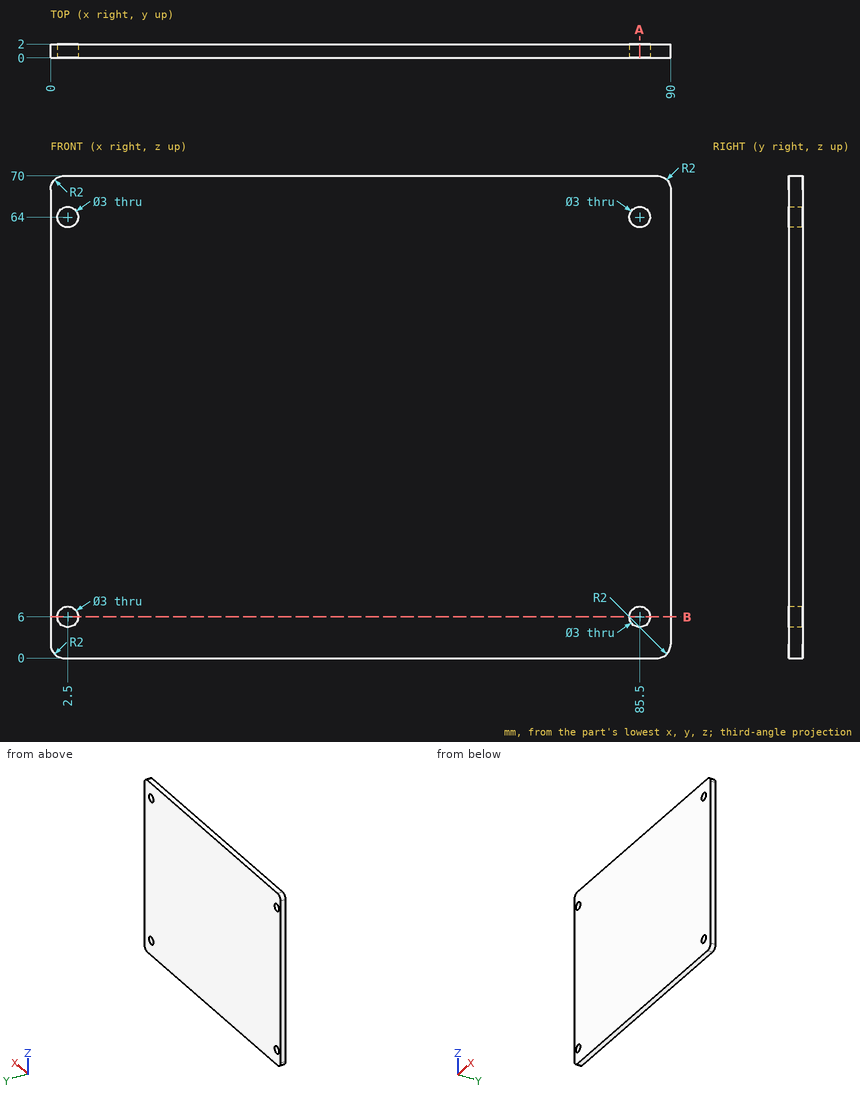
Geometry check sheet. Reference: drawing and pictorial views, mm from the part's lowest x, y, z. Give positions to 0.01 mm unless a question says otherwise; leave off trailing zeros. Order: outer loops, then holes, each group sorted by start corner. A loop starts at its lowest first (then second) coordinate and runs counter-clockwise, first axis right, second up. Notation, with made-up numbers: (59.5, -9.75) -> (73.5, -9.75) arc R27 ccw to (73.5, 13.25) -> close; hole circle Ø7 at (21, 72). An arc over 180 degrees is marked (long way). Use CSV: the item, a comma, the result in double quotes. Start each with the question number.
1) Sectioned sample at B-B, the plane z = 6. Record the boundary of the cut face in (x, y), plus the area to 3 significant figures.
2) Sectioned sample at A-A, the plane x = 85.5. Record the boundary of the cut face in (y, z).
3) Material ranges on line 1 (Z direction, x = 85.5, y = 1.3); line 2 (X direction, y = 1.35, z = 6), recorded low to high. Write a range as from..to.
Recorded:
1,outline,"(0, 0) -> (1, 0) -> (1, 2) -> (0, 2) -> close; (4, 0) -> (84, 0) -> (84, 2) -> (4, 2) -> close; (87, 0) -> (90, 0) -> (90, 2) -> (87, 2) -> close"
1,area,"168 mm2"
2,outline,"(0, 0) -> (2, 0) -> (2, 4.5) -> (0, 4.5) -> close; (0, 7.5) -> (2, 7.5) -> (2, 62.5) -> (0, 62.5) -> close; (0, 65.5) -> (2, 65.5) -> (2, 70) -> (0, 70) -> close"
3,line 1,"0..4.5, 7.5..62.5, 65.5..70"
3,line 2,"0..1, 4..84, 87..90"
